from build123d import *

# Parameters (mm, degrees)
BOSS_EXTRUDE1_DEPTH = 1.524


with BuildPart() as part:
    # Sketch1 → Boss-Extrude1 (new body)
    with BuildSketch(Plane.XY):
        with BuildLine():
            Line((73.000643508, 6.252619957), (70.027285358, 4.79070184))
            Line((70.027285358, 4.79070184), (69.354858347, 6.15833407))
            Line((69.354858347, 6.15833407), (72.727332666, 7.816486587))
            Line((72.727332666, 7.816486587), (71.978000913, 9.340533419))
            ThreePointArc((71.978000913, 9.340533419), (71.617545508, 9.701815407), (71.111637054, 9.768967549))
            ThreePointArc((71.111637054, 9.768967549), (66.728733529, 8.358005389), (62.788250891, 5.976146011))
            ThreePointArc((62.788250891, 5.976146011), (62.67763825, 5.871916038), (62.588919113, 5.748514423))
            ThreePointArc((62.588919113, 5.748514423), (62.289639081, 2.412826115), (64.660279583, 0.047144684))
            ThreePointArc((64.660279583, 0.047144684), (64.792973258, 0.011875), (64.929759758, 0))
            Line((64.929759758, 0), (73.399759676, 0))
            Line((73.399759676, 0), (73.399759676, -1.524))
            Line((73.399759676, -1.524), (64.804850415, -1.570364804))
            ThreePointArc((64.804850415, -1.570364804), (64.654260243, -1.585608721), (64.509301597, -1.629160622))
            ThreePointArc((64.509301597, -1.629160622), (62.262802552, -4.01311856), (62.588919113, -7.272514424))
            ThreePointArc((62.588919113, -7.272514424), (62.67763825, -7.395916038), (62.788250891, -7.500146011))
            ThreePointArc((62.788250891, -7.500146011), (66.728733529, -9.882005389), (71.111637054, -11.292967549))
            ThreePointArc((71.111637054, -11.292967549), (71.617545508, -11.225815407), (71.978000913, -10.864533419))
            Line((71.978000913, -10.864533419), (72.727332666, -9.340486587))
            Line((72.727332666, -9.340486587), (69.354858347, -7.68233407))
            Line((69.354858347, -7.68233407), (70.027285358, -6.31470184))
            Line((70.027285358, -6.31470184), (73.000643508, -7.776619957))
            ThreePointArc((73.000643508, -7.776619957), (73.406672693, -7.856097248), (73.797539642, -7.720452982))
            ThreePointArc((73.797539642, -7.720452982), (77.23855889, -5.019988283), (80.283555852, -1.879746802))
            ThreePointArc((80.283555852, -1.879746802), (80.451041219, -1.545581778), (80.447017019, -1.17181525))
            ThreePointArc((80.447017019, -1.17181525), (80.395843158, -0.762), (80.447017019, -0.35218475))
            ThreePointArc((80.447017019, -0.35218475), (80.451041219, 0.021581778), (80.283555852, 0.355746802))
            ThreePointArc((80.283555852, 0.355746802), (77.23855889, 3.495988283), (73.797539642, 6.196452982))
            ThreePointArc((73.797539642, 6.196452982), (73.406672693, 6.332097248), (73.000643508, 6.252619957))
        make_face()
    extrude(amount=BOSS_EXTRUDE1_DEPTH)


solid = part.part
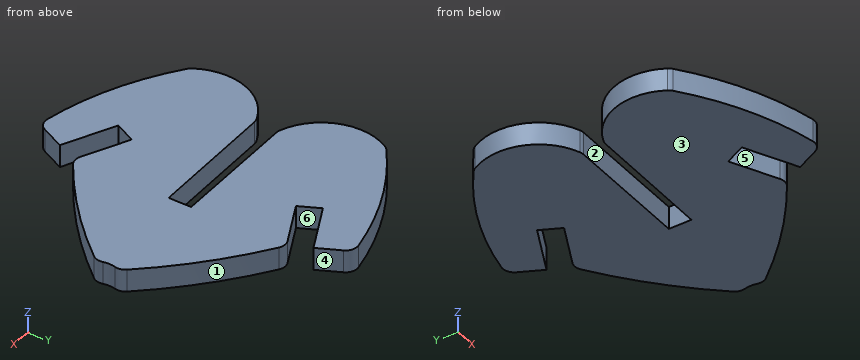
Here's how the part is built. I have some questions about the finished solid (model axes, mm). Face numbers are marked on the shaded views. A direction names the side the tool comes from. Coordinates: 2 decimals unless noted, no trailing zeros. Write each loop counter-clockwise with the first axis right and the second up, starting at its lowest first coordinate (ties: lowest second). Pieces come first, ordered by that corner, then holes.
Item 1: If I drill on line 1 (Y direction, x = 73, z = 0.7); line 2 (Y direction, x = 71, z = 1.05); line 3 (Y direction, x = 70.5, z = 0.7), over which ranges is the centre line in solid material (lowest first)?
Item 2: If we mould it in two halves opening along X, with no side actions, what happens to the marked faces 3, 4, 5 and 6? For each: +X half, -X half, draft (parallel to the pull), parting line (faces both ways), or undercut.
Item 3: Will these pins go through, and if not, where does the flat tip stop? pin 1 (2 mm diameter, centred on x = 75.5, y = 7, fed in from -Z); pin 2 (0.8 mm diameter, centred on y = -0.5, z = 0.5, fed in from -X); pin 3 (0.8 mm diameter, centred on x = 69, z = 0.5, fed in from -Y).
Item 4: I want a section at A-A on z = 0.75. Write out the boundary of the cut face in (x, y).
Item 5: I want a section at B-B on x = 72.5. Write out the boundary of the cut face in (y, z).
Item 6: On a 3-axis mill with a long thin cutter (end or side, diameter ignored), from which of +Z, -Z, +X, -X, +Y, -Y can I reach the whole of each face in a straight line? I mean the marked faces 1 and 2. Say none if no direction works.
Item 7: I want a section at D-D on y = -4. Write out the boundary of the cut face in (x, z).
Item 8: I want a section at C-C on y = -6.75. Write out the boundary of the cut face in (x, z), and give its area (3 significant figures).
Findings below:
1. line 1: y = -7.78 to -1.53, 0 to 6.25
1. line 2: y = -11.27 to -8.49, -6.79 to -1.54, 0 to 5.27, 6.97 to 9.75
1. line 3: y = -11.16 to -8.25, -6.55 to -1.54, 0 to 5.02, 6.72 to 9.64
2. face 3: draft
2. face 4: +X half
2. face 5: undercut
2. face 6: undercut
3. pin 1: passes through
3. pin 2: stops at x = 73.4
3. pin 3: stops at y = -10.87
4. outline: (62.59, -7.27) arc R0.79 ccw to (62.79, -7.5) arc R19.87 ccw to (71.11, -11.29) arc R0.79 ccw to (71.98, -10.86) - (72.73, -9.34) - (69.35, -7.68) - (70.03, -6.31) - (73, -7.78) arc R0.79 ccw to (73.8, -7.72) arc R32.33 ccw to (80.28, -1.88) arc R0.79 ccw to (80.45, -1.17) arc R1.67 cw to (80.45, -0.35) arc R0.79 ccw to (80.28, 0.36) arc R32.33 ccw to (73.8, 6.2) arc R0.79 ccw to (73, 6.25) - (70.03, 4.79) - (69.35, 6.16) - (72.73, 7.82) - (71.98, 9.34) arc R0.79 ccw to (71.11, 9.77) arc R19.87 ccw to (62.79, 5.98) arc R0.79 ccw to (62.59, 5.75) arc R3.95 ccw to (64.66, 0.05) arc R0.79 ccw to (64.93, 0) - (73.4, 0) - (73.4, -1.52) - (64.8, -1.57) arc R0.79 ccw to (64.51, -1.63) arc R3.95 ccw to start
5. outline: (-9.8, 0) - (-9.23, 0) - (-9.23, 1.52) - (-9.8, 1.52) - close; (-7.53, 0) - (-1.53, 0) - (-1.53, 1.52) - (-7.53, 1.52) - close; (0, 0) - (6.01, 0) - (6.01, 1.52) - (0, 1.52) - close; (7.7, 0) - (8.28, 0) - (8.28, 1.52) - (7.7, 1.52) - close
6. face 1: +Z, -Z, +X, +Y
6. face 2: +Z, -Z, -X
7. outline: (62.27, 0) - (78.32, 0) - (78.32, 1.52) - (62.27, 1.52) - close
8. outline: (62.33, 0) - (69.81, 0) - (69.81, 1.52) - (62.33, 1.52) - close; (70.91, 0) - (75.15, 0) - (75.15, 1.52) - (70.91, 1.52) - close
8. area: 17.9 mm2
